Verification items for this drawing (mm, ordinates from the low corner). A direction names the side the tool comes from. Round coordinates to 2 decimals unless told otherwise and drop trailing zeros. Loops run counter-clockwise (first coordinate to the right, second up) from the corner with the lowest first, then second, coordinate; pieces in that order, holes last. Notation, with made-up numbers: (34.5, -39.75) -> (72.5, -39.75) arc R25 cw to (72.5, -11.75) -> close; hole circle Ø2 at (79, 65). An arc over 180 degrees is marked (long way). One line per question, with ' | ' between items.
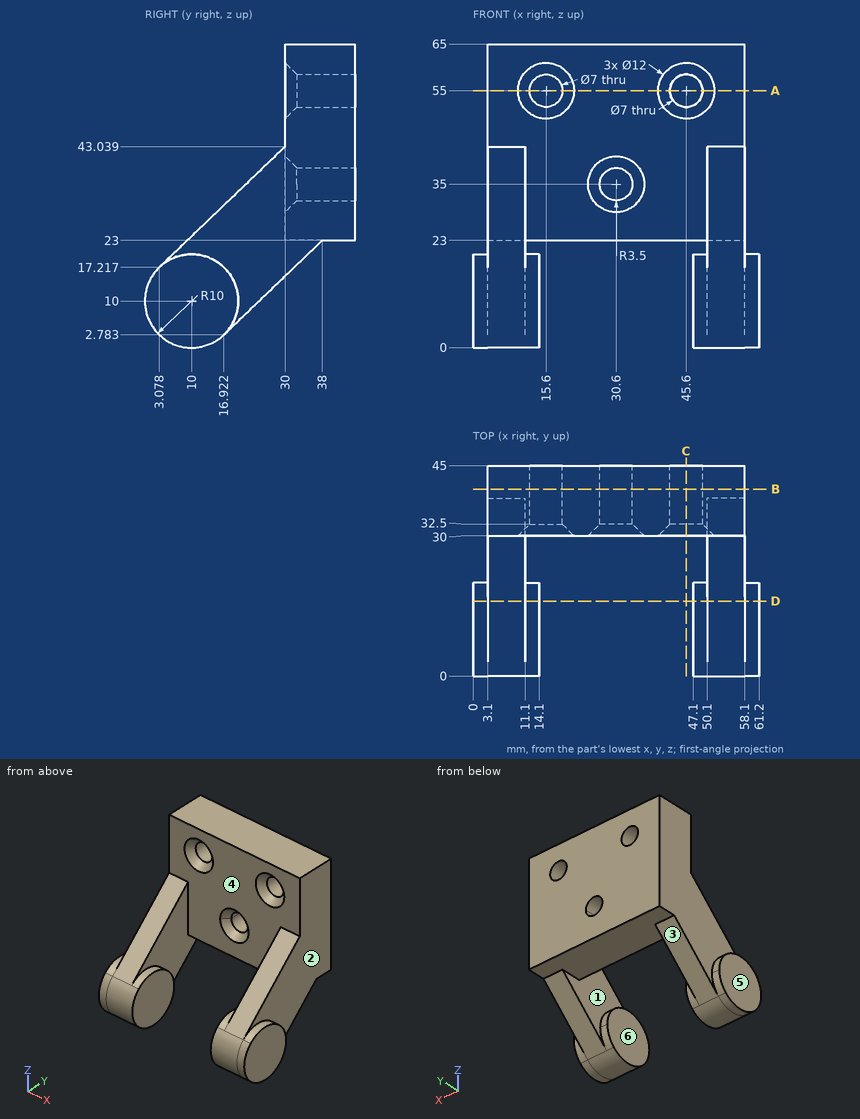
(1) Go/stop test with flat-tipped pins: pin 1 (12 mm diameter, centred on y = 33.5, z = 20, fed in from +X); pin 2 (12 mm diameter, centred on y = 29.5, z = 8.5, fed in from -X); pin 3 (3 mm diameter, centred on y = 32.5, z = 13, fed in from +X); pin 4 (10 mm diameter, centred on x = 19.5, z = 21.5, fed in from -Y). Record where each tip stops, or that it passes through.
Answer:
pin 1: stops at x = 58.1 | pin 2: stops at x = 3.1 | pin 3: passes through | pin 4: stops at y = 30
(2) Sectioned sample at D-D, the plane y = 16. Record the cut outline in (x, z), and give its area (3 significant figures).
Answer:
outline: (0, 2) -> (14.1, 2) -> (14.1, 18) -> (11.1, 18) -> (11.1, 29.61) -> (3.1, 29.61) -> (3.1, 18) -> (0, 18) -> close; (47.1, 2) -> (61.2, 2) -> (61.2, 18) -> (58.1, 18) -> (58.1, 29.61) -> (50.1, 29.61) -> (50.1, 18) -> (47.1, 18) -> close | area: 637 mm2
(3) Sectioned sample at A-A, the plane z = 55. Record the cut outline in (x, y).
Answer:
outline: (3.1, 30) -> (9.6, 30) -> (12.1, 32.5) -> (12.1, 45) -> (3.1, 45) -> close; (19.1, 32.5) -> (21.6, 30) -> (39.6, 30) -> (42.1, 32.5) -> (42.1, 45) -> (19.1, 45) -> close; (49.1, 32.5) -> (51.6, 30) -> (58.1, 30) -> (58.1, 45) -> (49.1, 45) -> close
(4) Sectioned sample at C-C, the plane x = 45.6. Record the cut outline in (y, z), and give its area (3 significant figures).
Answer:
outline: (30, 23) -> (45, 23) -> (45, 51.5) -> (32.5, 51.5) -> (30, 49) -> close; (30, 61) -> (32.5, 58.5) -> (45, 58.5) -> (45, 65) -> (30, 65) -> close | area: 519 mm2
(5) Mould release check, pull along X, two halves, no side actions. Record for the marked faces 1, 2 and 3: +X half, -X half, draft (parallel to the pull), parting line (faces both ways), or undercut.
Answer:
face 1: undercut | face 2: +X half | face 3: draft
(6) Sectioned sample at B-B, the plane y = 40. Record the cut outline in (x, z).
Answer:
outline: (3.1, 23) -> (58.1, 23) -> (58.1, 65) -> (3.1, 65) -> close; hole circle Ø7 at (15.6, 55); hole circle Ø7 at (30.6, 35); hole circle Ø7 at (45.6, 55)
(7) Set-up check for the marked faces 4, 5 and 6: record each of +Z, -Z, +X, -X, +Y, -Y from which the full face is reachable in a straight line by a thin tool's end or side.
Answer:
face 4: +Z, -Y | face 5: +Z, -Z, -X, +Y, -Y | face 6: +Z, -Z, +Y, -Y
(8) Scan lines: probe 1 along Z at (x, y) = (15.6, 39); probe 2 along X at (y, z) = (24.5, 33); probe 3 along Y at (x, z) = (45.5, 32). Record each from-to range of solid material in increasing order.
Answer:
probe 1: z = 23 to 51.5, 58.5 to 65 | probe 2: x = 3.1 to 11.1, 50.1 to 58.1 | probe 3: y = 30 to 45
